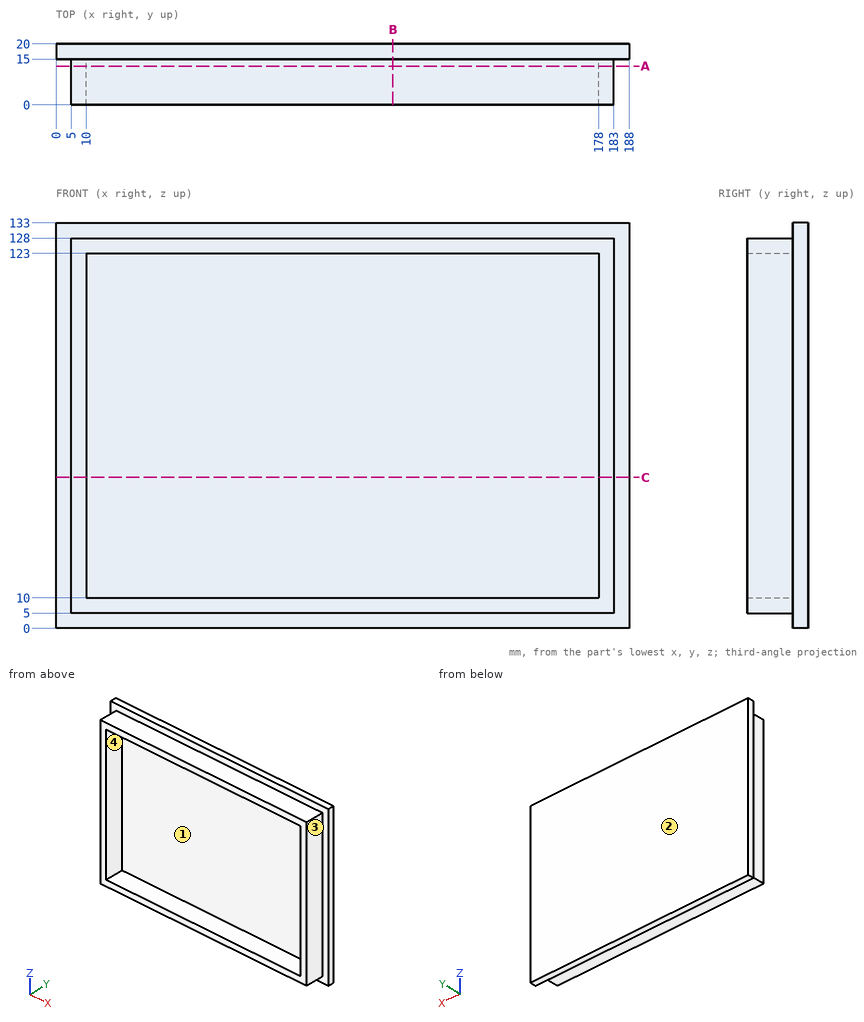
Geometry: see drawing. Coordinates: mm, zero at the bounding-box minimum. A direction names the side the tool comes from. Coordinates: 2 decimals unless noted, no trailing zeros. Order: outer loops, then holes, each group sorted by start corner. A loop starts at its lowest first (then second) coordinate and runs counter-clockwise, first axis right, second up. Notation, with made-up numbers: M 27,21 L 44,21 A28 ccw 44,55 Z; hole C 8.5,12 d10. An arc over 180 degrees is marked long. Write item = value, one per line. Start each with the question number.
(1) Section C-C on z = 49.5. Output: boundary loops of the cut face in (x, y), and give its area (3 significant figures).
(2) Section A-A on y = 12.75. Output: boundary loops of the cut face in (x, z).
(3) Section B-B on x = 110.5. Output: boundary loops of the cut face in (y, z).
(4) Pull-direction query (Z, two-part tool) for the marked faces 3 and 4; classes: released by +Z, released by -Z, zero draft, split by the parting line, or undercut.
(5) Line query: line 1 along Z through (x, y) = (158, 4.5); line 2 along X through (y, z) = (3.75, 115.5); line 3 along Y through (x, z) = (19, 63). Output: solid intervals per line, ascending. Write a range as [from, to].
(6) First-contact query: P1, Ø1.5, axis at x = 96, z = 31.5, coming from the -Y side; P2, Ø12, axis at x = 74, y = 4.5, coming from the +Z side; P3, Ø2, axis at y = 4, z = 28.5, coming from the -X side. Flat tips, straight axial feed; report the tip coordinate or a pass-through.
(7) Reachability of the marked faces 1 and 2 from +Z, -Z, +X, -X, +Y, -Y: full face, straight path, thin tool, end or side. Return the list, or none.
Result set:
q1.outline = M 0,15 L 5,15 L 5,0 L 10,0 L 10,15 L 178,15 L 178,0 L 183,0 L 183,15 L 188,15 L 188,20 L 0,20 Z
q1.area = 1,090 mm²
q2.outline = M 5,5 L 183,5 L 183,128 L 5,128 Z; hole M 10,10 L 178,10 L 178,123 L 10,123 Z
q3.outline = M 0,5 L 15,5 L 15,0 L 20,0 L 20,133 L 15,133 L 15,128 L 0,128 L 0,123 L 15,123 L 15,10 L 0,10 Z
q4.face_3 = zero draft
q4.face_4 = undercut
q5.line_1 = [5, 10], [123, 128]
q5.line_2 = [5, 10], [178, 183]
q5.line_3 = [15, 20]
q6.P1 = 15
q6.P2 = 128
q6.P3 = 5
q7.face_1 = -Y
q7.face_2 = +Z, -Z, +X, -X, +Y
